For this review, take the finished solid that the model builds, in its own axes (mm). Give positions to 0.01 mm unless a question says otherwise; leave off trailing zeros. Order: outer loops, then holes, each group sorted by start corner. A loop starts at its lowest first (then second) coordinate and runs counter-clockwise, first axis right, second up. Notation, with made-up numbers: M -35.5,37 L 23.5,37 A22 ccw 23.5,67 Z; hole C 56.5,4 d9. An arc over 180 degrees is marked long. Answer as CSV lines item,"result". Start each with the question number.
1. We need section B-B, the plane x = 10.5. Give the boundary of the cut face in (y, z).
2. For line 1 along X through (y, z) = (48.5, 2.7); line 2 along Y through (x, z) = (32.5, 2.45); line 3 along Y through (x, z) = (5.1, 2), list the stretches that pass through material, from the lowest coordinate up.
3. We need section C-C, the plane z = 1.3. State how many separate pieces and enclosed holes the cut face has, and give its area (3 significant figures).
4. Clearance check with flat-ended pins moving along their axes: P1, Ø0.8, axis at x = 37, z = 1, coming from the -Y side; P2, Ø1.4, axis at y = 55, z = 1.5, coming from the +X side; P3, Ø1.5, axis at x = 41.5, z = 1, coming from the +Y side; P4, Ø1.5, axis at x = 14.5, y = 15, coming from the -Z side. State where each tip first meets the part, or that it passes through.
5. We need section A-A, the plane y = 53. Give the boundary of the cut face in (x, z), and give its area (3 significant figures).
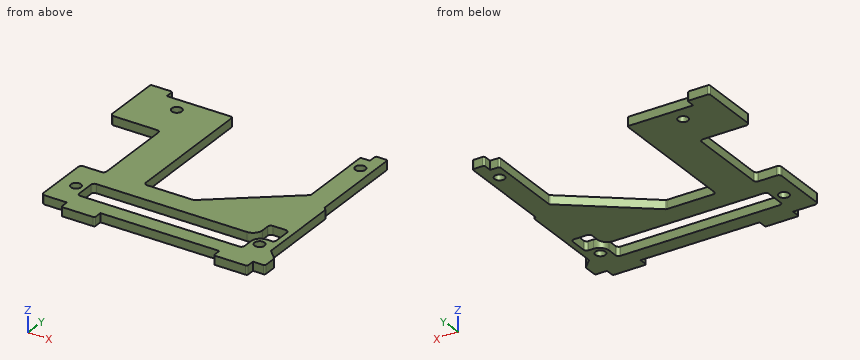
from build123d import *

# Parameters (mm, degrees)
SKETCH_R     = 1.6
PAD_DEPTH    = 2.8
POCKET_DEPTH = 2.801


with BuildPart() as part:
    # Sketch → Pad (new body)
    with BuildSketch(Plane.XY):
        with BuildLine():
            Line((1, 0), (8, 0))
            Line((8, 0), (8, -2.3))
            ThreePointArc((8, -2.3), (8.146447, -2.653553), (8.5, -2.8))
            Line((8.5, -2.8), (18.1, -2.8))
            ThreePointArc((18.1, -2.8), (18.453553, -2.653553), (18.6, -2.3))
            Line((18.6, -2.3), (18.6, 0))
            Line((18.6, 0), (56.2, 0))
            Line((56.2, 0), (56.2, -2.3))
            ThreePointArc((56.2, -2.3), (56.346447, -2.653553), (56.7, -2.8))
            Line((56.7, -2.8), (66.3, -2.8))
            ThreePointArc((66.3, -2.8), (66.653553, -2.653553), (66.8, -2.3))
            Line((66.8, -2.3), (66.8, 0))
            Line((66.8, 0), (70.1, 0))
            ThreePointArc((70.1, 0), (70.453553, 0.146447), (70.6, 0.5))
            Line((70.6, 0.5), (70.6, 4.292893))
            ThreePointArc((70.6, 4.292893), (70.56194, 4.484235), (70.453553, 4.646447))
            Line((70.453553, 4.646447), (67.6, 7.5))
            Line((67.6, 7.5), (67.6, 34))
            Line((67.6, 34), (66.8, 34.8))
            Line((66.8, 34.8), (66.8, 65))
            ThreePointArc((66.8, 65), (66.653553, 65.353553), (66.3, 65.5))
            Line((66.3, 65.5), (63.5, 65.5))
            ThreePointArc((63.5, 65.5), (63.146447, 65.353553), (63, 65))
            Line((63, 65), (63, 62.7))
            Line((63, 62.7), (60.5, 62.7))
            ThreePointArc((60.5, 62.7), (60.146447, 62.553553), (60, 62.2))
            Line((60, 62.2), (60, 38.8))
            ThreePointArc((59.807759, 38.405938), (59.949377, 38.580773), (60, 38.8))
            Line((59.807759, 38.405938), (35.607759, 19.505938))
            ThreePointArc((35.3, 19.4), (35.462741, 19.427226), (35.607759, 19.505938))
            Line((35.3, 19.4), (20.7, 19.4))
            ThreePointArc((19.7, 20.4), (19.992893, 19.692893), (20.7, 19.4))
            Line((19.7, 20.4), (19.7, 62.2))
            ThreePointArc((19.7, 62.2), (19.553553, 62.553553), (19.2, 62.7))
            Line((19.2, 62.7), (-1.2, 62.7))
            Line((-1.2, 62.7), (-1.2, 65))
            ThreePointArc((-1.2, 65), (-1.346447, 65.353553), (-1.7, 65.5))
            Line((-1.7, 65.5), (-7.6, 65.5))
            ThreePointArc((-7.6, 65.5), (-7.953553, 65.353553), (-8.1, 65))
            Line((-8.1, 65), (-8.1, 46.9))
            ThreePointArc((-8.1, 46.9), (-7.807107, 46.192893), (-7.1, 45.9))
            Line((-7.1, 45.9), (6.7, 45.9))
            ThreePointArc((7.7, 44.9), (7.407107, 45.607107), (6.7, 45.9))
            Line((7.7, 44.9), (7.7, 19.8))
            ThreePointArc((6.7, 18.8), (7.407107, 19.092893), (7.7, 19.8))
            Line((6.7, 18.8), (1, 18.8))
            ThreePointArc((1, 18.8), (0.292893, 18.507107), (0, 17.8))
            Line((0, 1), (0, 17.8))
            ThreePointArc((0, 1), (0.292893, 0.292893), (1, 0))
        make_face()
        with Locations((5.1, 57.9)):
            Circle(SKETCH_R, mode=Mode.SUBTRACT)
        with Locations((63.1, 57.9)):
            Circle(SKETCH_R, mode=Mode.SUBTRACT)
        with Locations((5.1, 8.9)):
            Circle(SKETCH_R, mode=Mode.SUBTRACT)
        with Locations((63.1, 8.9)):
            Circle(SKETCH_R, mode=Mode.SUBTRACT)
    extrude(amount=PAD_DEPTH)

    # Sketch001 → Pocket (cut, through all)
    with BuildSketch(Plane.XY):
        with BuildLine():
            Line((64.8, 19.1), (60.7, 19.1))
            ThreePointArc((60.7, 19.1), (59.992893, 18.807107), (59.7, 18.1))
            Line((59.7, 18.1), (59.7, 15.6))
            ThreePointArc((56.7, 12.6), (58.82132, 13.47868), (59.7, 15.6))
            Line((56.7, 12.6), (9.1, 12.6))
            ThreePointArc((9.1, 12.6), (8.392893, 12.307107), (8.1, 11.6))
            Line((8.1, 11.6), (8.1, 5.9))
            ThreePointArc((8.1, 5.9), (8.392893, 5.192893), (9.1, 4.9))
            Line((9.1, 4.9), (59.3, 4.9))
            ThreePointArc((59.3, 4.9), (60.007107, 5.192893), (60.3, 5.9))
            Line((60.3, 5.9), (60.3, 9))
            ThreePointArc((63.3, 12), (61.17868, 11.12132), (60.3, 9))
            Line((63.3, 12), (64.8, 12))
            ThreePointArc((64.8, 12), (65.507107, 12.292893), (65.8, 13))
            Line((65.8, 13), (65.8, 18.1))
            ThreePointArc((65.8, 18.1), (65.507107, 18.807107), (64.8, 19.1))
        make_face()
    extrude(amount=POCKET_DEPTH, mode=Mode.SUBTRACT)


solid = part.part
Result set:
1,outline,"M -2.8,0 L 4.9,0 L 4.9,2.8 L -2.8,2.8 Z; M 12.6,0 L 62.7,0 L 62.7,2.8 L 12.6,2.8 Z"
2,line 1,"-8.1 to 19.7, 60 to 66.8"
2,line 2,"0 to 4.9, 12.6 to 19.4"
2,line 3,"0 to 7.3, 10.5 to 18.8, 45.9 to 56.3, 59.5 to 62.7"
3,separate pieces,"1"
3,enclosed holes,"5"
3,area,"2,260 mm2"
4,P1,"y = 0"
4,P2,"x = 66.8"
4,P3,"y = 24.69"
4,P4,"z = 0"
5,outline,"M -8.1,0 L 19.7,0 L 19.7,2.8 L -8.1,2.8 Z; M 60,0 L 66.8,0 L 66.8,2.8 L 60,2.8 Z"
5,area,"96.9 mm2"
